from build123d import *

# Parameters (mm, degrees)
F0_W     = 28.448
F0_H     = 31.75
F1_DEPTH = 73.406
F3_DEPTH = 7.874
F5_W     = 6.35
F5_H     = 28.448
F6_DEPTH = 4.826
F7_W     = 6.35
F7_H     = 28.448
F8_DEPTH = 4.826


with BuildPart() as f1:
    # F0 (on Right) → F1 (new body)
    with BuildSketch(Plane.YZ):
        Rectangle(F0_W, F0_H)
    extrude(amount=F1_DEPTH)

    # F2 (on Front) → F3 (join, symmetric)
    with BuildSketch(Plane.XZ):
        Polygon((0, -44.323), (104.648, -44.323), (76.2, -15.875), (73.406, -15.875), (0, -15.875), align=None)
        with BuildLine():
            ThreePointArc((30.226, -35.687), (24.638, -30.099), (30.226, -24.511))
            Line((30.226, -24.511), (54.102, -24.511))
            ThreePointArc((54.102, -24.511), (58.053313, -26.147687), (59.69, -30.099))
            ThreePointArc((59.69, -30.099), (58.053313, -34.050313), (54.102, -35.687))
            Line((54.102, -35.687), (30.226, -35.687))
        make_face(mode=Mode.SUBTRACT)
        Polygon((0, 15.875), (73.406, 15.875), (76.2, 15.875), (104.648, 44.323), (0, 44.323), align=None)
        with BuildLine():
            ThreePointArc((30.226, 24.511), (24.638, 30.099), (30.226, 35.687))
            Line((30.226, 35.687), (54.102, 35.687))
            ThreePointArc((54.102, 35.687), (58.053313, 34.050313), (59.69, 30.099))
            ThreePointArc((59.69, 30.099), (58.053313, 26.147687), (54.102, 24.511))
            Line((54.102, 24.511), (30.226, 24.511))
        make_face(mode=Mode.SUBTRACT)
    extrude(amount=F3_DEPTH, both=True)

    # F5 (on face) → F6 (cut)
    with BuildSketch(Plane.XZ.offset(7.874)):
        with Locations((3.175, 30.099)):
            Rectangle(F5_W, F5_H)
    extrude(amount=-F6_DEPTH, mode=Mode.SUBTRACT)

    # F7 (on face) → F8 (cut)
    with BuildSketch(Plane.XZ.offset(7.874)):
        with Locations((3.175, -30.099)):
            Rectangle(F7_W, F7_H)
    extrude(amount=-F8_DEPTH, mode=Mode.SUBTRACT)


solid = f1.part
Build history of the part. All positions in model axes, mm. A direction names the side the tool comes from. Give positions to 0.01 mm unless a question says otherwise; leave off trailing zeros. Loops run counter-clockwise (first coordinate to the right, second up) from the corner with the lowest first, then second, coordinate; pieces in that order, holes last. Notation, with made-up numbers: (64, 37) - (103, 37) arc R21 cw to (103, 48) - close; hole circle Ø11 at (-6.5, 41). An arc over 180 degrees is marked (long way). Write item = value, one per line. Start each with the question number.
1) Band-saw the part on D-D on y = -1.25. Give the cut face in (x, z) (3 decimals).
2) Band-saw the part on C-C on x = 96. Give the cut face in (y, z) (3 decimals).
3) Probe probe 1 along Z at (x, y) = (41.5, -5.75); probe 2 along Z at (x, y) = (45, 10.25) (3 decimals); probe 3 along Y at (x, z) = (17.5, 30.5). List the from-to ranges inside material, lowest first. Write a range as from..to.
4) Drop flat-ended pins along their axis: pin 1 Ø10 at (x, z) = (16.5, 34) entering from +Y; pin 2 Ø3 at (x, y) = (19.5, 9.5) entering from +Z (3 decimals); pin 3 Ø8.5 at (x, z) = (72.5, -23) entering from -Y. Give the stop position or say it passes through.
5) Tool access for faces 4 (the flat face through (42, 0, 35.687)), 5 (the flat face through (36, 11, 15.875)), 6 (the flat face through (90.225, -0.11, 29.9)): list every direction of +Z, -Z, +X, -X, +Y, -Y with a clear straight run to the whole face (end or side of a thin tool).
6) Band-saw the part on B-B on x = 37. Give the cut face in (y, z) (3 decimals), plus the area to 3 significant figures.
7) Pull direction X, two halves, no side cores. Call faces 1 (the cylindrical face through (24.64, -0.11, 29.98)), 2 (the flat face through (6.35, -5, 30)), 3 (the flat face through (36, 11, -15.875)): +X half, -X half, draft (parallel to the pull), parting line (faces both ways), or undercut.
8) Band-saw the part on A-A on y = -6.5. Give the cut face in (x, z) (3 decimals).
Final values:
q1.outline = (0, -44.323) - (104.648, -44.323) - (76.2, -15.875) - (73.406, -15.875) - (73.406, 15.875) - (76.2, 15.875) - (104.648, 44.323) - (0, 44.323) - close; hole (30.226, -35.687) - (54.102, -35.687) arc R5.588 ccw to (59.69, -30.099) arc R5.588 ccw to (54.102, -24.511) - (30.226, -24.511) arc R5.588 ccw to start; hole (30.226, 24.511) - (54.102, 24.511) arc R5.588 ccw to (59.69, 30.099) arc R5.588 ccw to (54.102, 35.687) - (30.226, 35.687) arc R5.588 ccw to start
q2.outline = (-7.874, -44.323) - (7.874, -44.323) - (7.874, -35.675) - (-7.874, -35.675) - close; (-7.874, 35.675) - (7.874, 35.675) - (7.874, 44.323) - (-7.874, 44.323) - close
q3.probe_1 = -44.32..-35.69, -24.51..24.51, 35.69..44.32
q3.probe_2 = -15.875..15.875
q3.probe_3 = -7.87..7.87
q4.pin_1 = 7.87
q4.pin_2 = 15.875
q4.pin_3 = -7.87
q5.face_4 = +Y, -Y
q5.face_5 = +Z, +X, -X, +Y
q5.face_6 = +X, +Y, -Y
q6.outline = (-14.224, -15.875) - (-7.874, -15.875) - (-7.874, -24.511) - (7.874, -24.511) - (7.874, -15.875) - (14.224, -15.875) - (14.224, 15.875) - (7.874, 15.875) - (7.874, 24.511) - (-7.874, 24.511) - (-7.874, 15.875) - (-14.224, 15.875) - close; (-7.874, -44.323) - (7.874, -44.323) - (7.874, -35.687) - (-7.874, -35.687) - close; (-7.874, 35.687) - (7.874, 35.687) - (7.874, 44.323) - (-7.874, 44.323) - close
q6.area = 1,450 mm²
q7.face_1 = undercut
q7.face_2 = -X half
q7.face_3 = draft
q8.outline = (0, -15.875) - (6.35, -15.875) - (6.35, -44.323) - (104.648, -44.323) - (76.2, -15.875) - (73.406, -15.875) - (73.406, 15.875) - (76.2, 15.875) - (104.648, 44.323) - (6.35, 44.323) - (6.35, 15.875) - (0, 15.875) - close; hole (30.226, -35.687) - (54.102, -35.687) arc R5.588 ccw to (59.69, -30.099) arc R5.588 ccw to (54.102, -24.511) - (30.226, -24.511) arc R5.588 ccw to start; hole (30.226, 24.511) - (54.102, 24.511) arc R5.588 ccw to (59.69, 30.099) arc R5.588 ccw to (54.102, 35.687) - (30.226, 35.687) arc R5.588 ccw to start
